```python
from build123d import *

# Parameters (mm, degrees)
SALIENTE_EXTRUIR1_DEPTH    = 30
CORTAR_EXTRUIR1_DEPTH      = 15
CORTAR_EXTRUIR1_DEPTH_BACK = 41
CROQUIS2_R                 = 1.6
CROQUIS3_R                 = 2.9
CORTAR_EXTRUIR2_DEPTH      = 3.2
SKETCH1_R                  = 0.661549992
CUT_EXTRUDE1_DEPTH         = 0.4


with BuildPart() as part:
    # Croquis1 → Saliente-Extruir1 (new body)
    with BuildSketch(Plane.XY):
        Polygon((-21, 0), (-21, 27), (-13, 27), (-13, 3), (13, 3), (13, 27), (21, 27), (21, 0), align=None)
    extrude(amount=SALIENTE_EXTRUIR1_DEPTH)

    # Croquis2 → Cortar-Extruir1 (cut, two sides: drawn at the far end of the back side and taken through both)
    with BuildSketch(Plane.XZ.offset(-CORTAR_EXTRUIR1_DEPTH_BACK)):
        with Locations(Location((-17, 15, 0), (0, 0, 90))):
            Circle(CROQUIS2_R)
        with Locations(Location((17, 15, 0), (0, 0, 90))):
            Circle(CROQUIS2_R)
    extrude(amount=CORTAR_EXTRUIR1_DEPTH + CORTAR_EXTRUIR1_DEPTH_BACK, mode=Mode.SUBTRACT)

    # Croquis3 → Cortar-Extruir2 (cut)
    with BuildSketch(Plane.XZ):
        with Locations(Location((-17, 15, 0), (0, 0, 270))):
            Circle(CROQUIS3_R)
        with Locations(Location((17, 15, 0), (0, 0, 90))):
            Circle(CROQUIS3_R)
    extrude(amount=-CORTAR_EXTRUIR2_DEPTH, mode=Mode.SUBTRACT)

    # Sketch1 → Cut-Extrude1 (cut)
    # profile 1 of 7: a face of its own
    with BuildSketch(Plane.XZ):
        with BuildLine():
            Line((-5.935999793, 6.438605572), (9.678181575, 6.438605572))
            add(Edge.make_bspline(
                [(9.678181575, 6.438605572), (10.524299676, 6.453092153), (10.536716692, 7.227891763)],
                knots=[0, 0, 0, 1, 1, 1], degree=2))
            Line((10.536716692, 7.227891763), (10.536716692, 20.957100846))
            add(Edge.make_bspline(
                [(9.678181575, 22.106217079), (10.162482833, 22.073196538), (10.536716692, 21.695427507), (10.536716692, 20.957100846)],
                knots=[0, 0, 0, 0, 1, 1, 1, 1], degree=3))
            Line((9.678181575, 22.106217079), (9.004561714, 22.106217079))
            add(Edge.make_bspline(
                [(8.312539005, 20.630919436), (8.286013306, 22.128234394), (8.338307263, 22.106217079), (9.004561714, 22.106217079)],
                knots=[0, 0, 0, 0, 1, 1, 1, 1], degree=3))
            add(Edge.make_bspline(
                [(8.867643901, 19.868961385), (8.878593238, 20.486835473), (8.312539005, 20.630919436)],
                knots=[0, 0, 0, 1, 1, 1], degree=2))
            Line((8.867643901, 19.868961385), (8.867643901, 9.082596351))
            add(Edge.make_bspline(
                [(7.931444331, 8.073576195), (8.599546043, 8.102198014), (8.867643901, 8.329896708), (8.867643901, 9.082596351)],
                knots=[0, 0, 0, 0, 1, 1, 1, 1], degree=3))
            Line((7.931444331, 8.073576195), (-4.462187712, 8.073576195))
            add(Edge.make_bspline(
                [(-5.467904846, 9.082596351), (-5.433709159, 8.449976132), (-5.30844888, 8.073576195), (-4.462187712, 8.073576195)],
                knots=[0, 0, 0, 0, 1, 1, 1, 1], degree=3))
            Line((-5.467904846, 9.082596351), (-5.467904846, 16.225240488))
            add(Edge.make_bspline(
                [(-6.227323907, 16.964134709), (-5.679994854, 16.964134709), (-5.467904846, 16.719544079), (-5.467904846, 16.225240488)],
                knots=[0, 0, 0, 0, 1, 1, 1, 1], degree=3))
            add(Edge.make_bspline(
                [(-7.060451344, 16.225240488), (-7.033250732, 16.738079235), (-6.945687764, 17.041102265), (-6.227323907, 16.964134709)],
                knots=[0, 0, 0, 0, 1, 1, 1, 1], degree=3))
            Line((-7.060451344, 16.225240488), (-7.060451344, 7.629208643))
            add(Edge.make_bspline(
                [(-5.935999793, 6.438605572), (-6.811453061, 6.382227451), (-7.096596098, 6.700746565), (-7.060451344, 7.629208643)],
                knots=[0, 0, 0, 0, 1, 1, 1, 1], degree=3))
        make_face()
    # profile 2 of 7: a face of its own
    with BuildSketch(Plane.XZ):
        with BuildLine():
            Line((-1.522038325, 11.057965372), (-3.304487637, 9.883355918))
            Line((-3.304487637, 9.883355918), (-3.95725526, 10.532266036))
            Line((-3.95725526, 10.532266036), (-2.69664778, 12.281859139))
            add(Edge.make_bspline(
                [(-2.69664778, 12.281859139), (-2.296419712, 12.30894865), (-1.901088431, 12.60910176)],
                knots=[0, 0, 0, 1, 1, 1], degree=2))
            Line((-1.901088431, 12.60910176), (-0.072061062, 14.43812913))
            Line((-0.072061062, 14.43812913), (0.678700134, 13.69714151))
            Line((0.678700134, 13.69714151), (-1.199414528, 11.794254647))
            add(Edge.make_bspline(
                [(-1.522038325, 11.057965372), (-1.526686537, 11.364992788), (-1.400661149, 11.590353596), (-1.199414528, 11.794254647)],
                knots=[0, 0, 0, 0, 1, 1, 1, 1], degree=3))
        make_face()
    # profile 3 of 7: a face of its own
    with BuildSketch(Plane.XZ):
        with BuildLine():
            Line((-0.354442309, 15.390176677), (5.412555572, 9.698254849))
            add(Edge.make_bspline(
                [(5.412555572, 9.698254849), (5.928798687, 9.302057302), (6.700610258, 9.391128714), (7.125727085, 9.883355918)],
                knots=[0, 0, 0, 0, 1, 1, 1, 1], degree=3))
            add(Edge.make_bspline(
                [(7.125727085, 9.883355918), (7.934302129, 10.799871296), (6.977240411, 11.794254647)],
                knots=[0, 0, 0, 1, 1, 1], degree=2))
            Line((6.977240411, 11.794254647), (1.303415875, 17.468079182))
            add(Edge.make_bspline(
                [(1.303415875, 17.468079182), (1.911666945, 20.540477103), (-1.10270103, 21.574939106), (-2.42824136, 20.752545127)],
                knots=[0, 0, 0, 0, 1, 1, 1, 1], degree=3))
            Line((-2.42824136, 20.752545127), (-0.694584651, 19.041457544))
            Line((-0.694584651, 19.041457544), (-1.366070433, 17.845234527))
            Line((-1.366070433, 17.845234527), (-2.405054872, 17.553329375))
            Line((-2.405054872, 17.553329375), (-4.123067785, 19.248976817))
            add(Edge.make_bspline(
                [(-0.354442309, 15.390176677), (-3.400230967, 14.629724328), (-5.142448484, 17.119603802), (-4.123067785, 19.248976817)],
                knots=[0, 0, 0, 0, 1, 1, 1, 1], degree=3))
        make_face()
        with Locations(Location((6.13875523, 10.776625251, 0), (0, 0, 270))):
            Circle(SKETCH1_R, mode=Mode.SUBTRACT)
    # profile 4 of 7: a face of its own
    with BuildSketch(Plane.XZ):
        with BuildLine():
            Line((3.89207141, 15.458279189), (1.891941088, 17.586897539))
            Line((1.891941088, 17.586897539), (5.230965028, 20.957100846))
            add(Edge.make_bspline(
                [(5.230965028, 20.957100846), (5.555451632, 21.309870343), (6.660184694, 21.36409952), (7.269640603, 20.523170445)],
                knots=[0, 0, 0, 0, 1, 1, 1, 1], degree=3))
            add(Edge.make_bspline(
                [(7.242774573, 18.701199897), (8.073193496, 19.568863686), (7.269640603, 20.523170445)],
                knots=[0, 0, 0, 1, 1, 1], degree=2))
            Line((7.242774573, 18.701199897), (3.89207141, 15.458279189))
        make_face()
        Polygon((3.839024866, 17.163144155), (4.259148948, 16.746906842), (6.762194587, 19.273325593), (6.342070505, 19.689562906), align=None, mode=Mode.SUBTRACT)
        Polygon((3.102284891, 17.893068195), (3.522408973, 17.476830882), (6.025454613, 20.003249633), (5.60533053, 20.419486946), align=None, mode=Mode.SUBTRACT)
    # profile 5 of 7: a face of its own
    with BuildSketch(Plane.XZ):
        with BuildLine():
            add(Edge.make_bspline(
                [(-7.099579962, 18.308936967), (-6.944184766, 19.799579775), (-5.756766751, 20.990125682), (-4.011121589, 21.166157127)],
                knots=[0, 0, 0, 0, 1, 1, 1, 1], degree=3))
            add(Edge.make_bspline(
                [(-4.011121589, 21.166157127), (-3.833143245, 21.190875028), (-3.641894385, 21.375340953), (-3.624888541, 21.60783322)],
                knots=[0, 0, 0, 0, 1, 1, 1, 1], degree=3))
            add(Edge.make_bspline(
                [(-3.624888541, 21.60783322), (-3.639467746, 21.893086016), (-3.884725351, 22.173601101), (-4.195925218, 22.143963019)],
                knots=[0, 0, 0, 0, 1, 1, 1, 1], degree=3))
            add(Edge.make_bspline(
                [(-8.06346903, 18.701199897), (-7.725118315, 20.514418332), (-5.974799785, 22.083491135), (-4.195925218, 22.143963019)],
                knots=[0, 0, 0, 0, 1, 1, 1, 1], degree=3))
            add(Edge.make_bspline(
                [(-7.614023361, 17.927066284), (-8.122682955, 17.975749279), (-8.06346903, 18.701199897)],
                knots=[0, 0, 0, 1, 1, 1], degree=2))
            add(Edge.make_bspline(
                [(-7.099579962, 18.308936967), (-7.183532259, 17.914926879), (-7.614023361, 17.927066284)],
                knots=[0, 0, 0, 1, 1, 1], degree=2))
        make_face()
    # profile 6 of 7: a face of its own
    with BuildSketch(Plane.XZ):
        with BuildLine():
            add(Edge.make_bspline(
                [(-9.319053754, 18.411393731), (-9.333101087, 19.560108027), (-7.895947649, 23.219067723), (-3.95725526, 23.325518869)],
                knots=[0, 0, 0, 0, 1, 1, 1, 1], degree=3))
            add(Edge.make_bspline(
                [(-3.95725526, 23.325518869), (-3.779276916, 23.35023677), (-3.597859082, 23.595665467), (-3.624888541, 23.776531501)],
                knots=[0, 0, 0, 0, 1, 1, 1, 1], degree=3))
            add(Edge.make_bspline(
                [(-3.624888541, 23.776531501), (-3.639467746, 24.061784297), (-3.884725351, 24.317135086), (-4.195925218, 24.287497003)],
                knots=[0, 0, 0, 0, 1, 1, 1, 1], degree=3))
            add(Edge.make_bspline(
                [(-10.243657996, 18.701199897), (-10.182828773, 20.346306567), (-8.409956491, 24.044181671), (-4.195925218, 24.287497003)],
                knots=[0, 0, 0, 0, 1, 1, 1, 1], degree=3))
            add(Edge.make_bspline(
                [(-9.805687565, 17.927066284), (-10.31434716, 17.975749279), (-10.243657996, 18.701199897)],
                knots=[0, 0, 0, 1, 1, 1], degree=2))
            add(Edge.make_bspline(
                [(-9.319053754, 18.411393731), (-9.375196464, 17.914926879), (-9.805687565, 17.927066284)],
                knots=[0, 0, 0, 1, 1, 1], degree=2))
        make_face()
    # profile 7 of 7: a face of its own
    with BuildSketch(Plane.XZ):
        with BuildLine():
            add(Edge.make_bspline(
                [(-11.523144368, 18.395379414), (-11.040898376, 22.612315512), (-7.900523453, 25.441163991), (-3.961831064, 25.547615136)],
                knots=[0, 0, 0, 0, 1, 1, 1, 1], degree=3))
            add(Edge.make_bspline(
                [(-3.961831064, 25.547615136), (-3.783852719, 25.572333037), (-3.602434885, 25.817761734), (-3.629464345, 25.998627769)],
                knots=[0, 0, 0, 0, 1, 1, 1, 1], degree=3))
            add(Edge.make_bspline(
                [(-3.629464345, 25.998627769), (-3.644043549, 26.283880564), (-3.889301155, 26.539231353), (-4.200501022, 26.50959327)],
                knots=[0, 0, 0, 0, 1, 1, 1, 1], degree=3))
            add(Edge.make_bspline(
                [(-12.44774861, 18.68518558), (-12.386919387, 20.33029225), (-10.637820975, 26.082784436), (-4.200501022, 26.50959327)],
                knots=[0, 0, 0, 0, 1, 1, 1, 1], degree=3))
            add(Edge.make_bspline(
                [(-12.00977818, 17.911051966), (-12.518437774, 17.959734961), (-12.44774861, 18.68518558)],
                knots=[0, 0, 0, 1, 1, 1], degree=2))
            add(Edge.make_bspline(
                [(-11.523144368, 18.395379414), (-11.579287078, 17.898912561), (-12.00977818, 17.911051966)],
                knots=[0, 0, 0, 1, 1, 1], degree=2))
        make_face()
    extrude(amount=-CUT_EXTRUDE1_DEPTH, mode=Mode.SUBTRACT)


solid = part.part
```
Geometry check sheet. Reference: the model listing, model coordinates, mm. A direction names the side the tool comes from. Give positions to 0.01 mm unless a question says otherwise; leave off trailing zeros. Loops run counter-clockwise (first coordinate to the right, second up) from the corner with the lowest first, then second, coordinate; pieces in that order, holes last. Notation, with made-up numbers: M -15.5,68 L 35.5,68 A10 ccw 35.5,85 Z; hole C -21.75,16 d11. An arc over 180 degrees is marked long. Write item = value, one per line. Start each with the question number.
1. Section check B-B, the plane x = -17. Enter the section's corners in (y, z), plus the area to 3 significant figures.
2. Go/stop test with flat-tipped pins: P1, Ø6, axis at x = 9.5, z = 5.5, coming from the +Y side; P2, Ø1.9, axis at x = -17, z = 15, coming from the +Y side. Record where each tip stops, or that it passes through.
3. Tool access check on faces 1 (the face through (4.37, 0.2, 19.17)), 2 (the face through (0, 0, 11)). Record the directions out of +Z, -Z, +X, -X, +Y, -Y that give a thin tool (end or side, any length) a straight path to the whole face; none if there is none.
4. Section check A-A, the plane y = 16. Enter the section's corners in (x, z).
5. Draft check along Z on faces 3 (the face through (-1, 0.2, 13.51)), 4 (the face through (4.6, 0, 19.1)), 5 (the face through (15.92, 15.27, 13.82)). Enter one of: +Z half, -Z half, draft (parallel to the pull), parting line (faces both ways), or undercut.
6. Thickness scan on probe 1 along X at (y, z) = (10.75, 15); probe 2 along X at (y, z) = (4, 11); probe 3 along X at (y, z) = (1.25, 17.5). Record the ranges inside material, lowest first.
Values follow:
q1.outline = M 0,0 L 27,0 L 27,13.4 L 3.2,13.4 L 3.2,12.1 L 0,12.1 Z; M 0,17.9 L 3.2,17.9 L 3.2,16.6 L 27,16.6 L 27,30 L 0,30 Z
q1.area = 715 mm^2
q2.P1 = 3
q2.P2 = through
q3.face_1 = -Y
q3.face_2 = +Z, -Z, +X, -X, -Y
q4.outline = M -21,0 L -13,0 L -13,30 L -21,30 Z; M 13,0 L 21,0 L 21,30 L 13,30 Z; hole C -17,15 d3.2; hole C 17,15 d3.2
q5.face_3 = undercut
q5.face_4 = draft
q5.face_5 = undercut
q6.probe_1 = -21 to -18.6, -15.4 to -13, 13 to 15.4, 18.6 to 21
q6.probe_2 = -21 to -13, 13 to 21
q6.probe_3 = -21 to -18.47, -15.53 to 15.53, 18.47 to 21
